from build123d import *

# Parameters (mm, degrees)
SKETCH1_W           = 38.481
SKETCH1_H           = 38.481
BOSS_EXTRUDE1_DEPTH = 12.573
SKETCH2_W           = 36.703
SKETCH2_H           = 36.703
CUT_EXTRUDE1_DEPTH  = 56.853872301
SKETCH3_R           = 2.4765
CUT_EXTRUDE2_DEPTH  = 55.644102143


with BuildPart() as part:
    # Sketch1 → Boss-Extrude1 (new body)
    with BuildSketch(Plane.XY):
        with Locations((19.2405, 19.2405)):
            Rectangle(SKETCH1_W, SKETCH1_H)
    extrude(amount=BOSS_EXTRUDE1_DEPTH)

    # Sketch2 → Cut-Extrude1 (cut, through all)
    with BuildSketch(Plane.XY.offset(12.573)):
        with Locations((18.3515, 20.1295)):
            Rectangle(SKETCH2_W, SKETCH2_H)
    extrude(amount=-CUT_EXTRUDE1_DEPTH, mode=Mode.SUBTRACT)

    # Sketch3 → Cut-Extrude2 (cut, through all)
    with BuildSketch(Plane.ZY.offset(-36.703)):
        with Locations(Location((6.2865, 12.6365, 0), (0, 0, 270))):
            Circle(SKETCH3_R)
        with Locations(Location((6.2865, 30.5435, 0), (0, 0, 270))):
            Circle(SKETCH3_R)
    cut_extrude2 = extrude(amount=-CUT_EXTRUDE2_DEPTH, mode=Mode.SUBTRACT)

    # Mirror1: Cut-Extrude2 across plane
    add(cut_extrude2.mirror(Plane(origin=(19.2405, 19.2405, 0), x_dir=(0, 0, 1), z_dir=(0.7071067811865389, 0.7071067811865561, 0))), mode=Mode.SUBTRACT)


solid = part.part
Verification items for the finished model (mm, model axes). A direction names the side the tool comes from. Coordinates: 2 decimals unless noted, no trailing zeros. Order: outer loops, then holes, each group sorted by start corner. A loop starts at its lowest first (then second) coordinate and runs counter-clockwise, first axis right, second up. Notation, with made-up numbers: (30, -0.75) -> (83, -0.75) arc R14 cw to (83, 16.25) -> close; hole circle Ø2 at (-5, 6.25). An arc over 180 degrees is marked (long way). Use CSV: the item, a comma, the result in double quotes. Start each with the question number.
Q1. Tool access check on faces 5 (the flat face through (18, 1.778, 6)), 6 (the cylindrical face through (37.58, 15.11, 6.4)). Record the directions out of +Z, -Z, +X, -X, +Y, -Y that give a thin tool (end or side, any length) a straight path to the whole face; none if there is none.
Q2. Thickness scan on line 1 along X through (y, z) = (10, 5.75); line 2 along Y through (x, z) = (23, 9.25). Record the ranges inside material, lowest first.
Q3. Section check B-B, the plane x = 8.5. Record the cut outline in (y, z), and give its area (3 significant figures).
Q4. Depth check by flat-ended pin: P1, Ø3, axis at x = 28, z = 9, coming from the +Y side. Enter the tip coordinate at first touch or a pass-through.
Q5. Section check C-C, the plane y = 31.5. Record the cut outline in (x, z), and give its area (3 significant figures).
Q6. Draft check along X on faces 1 (the flat face through (19, 0, 6)), 2 (the flat face through (38.481, 19, 6)), 3 (the cylindrical face through (5.97, 0.9, 4.78)), 4 (the cylindrical face through (28.207, 0.901, 7.03)). Enter one of: +X half, -X half, draft (parallel to the pull), parting line (faces both ways), or undercut.
Q7. Section check A-A, the plane z = 7. Record the cut outline in (x, y) (3 decimals), and give its area (3 significant figures).
Q8. Section check D-D, the plane z = 2.75. Record the cut outline in (x, y).
Returned:
1,face 5,"+Z, -Z, -X, +Y"
1,face 6,"+X, -X"
2,line 1,"x = 36.7 to 38.48"
2,line 2,"y = 0 to 1.78"
3,outline,"(0, 0) -> (1.78, 0) -> (1.78, 3.87) -> (0, 3.87) -> close; (0, 8.7) -> (1.78, 8.7) -> (1.78, 12.57) -> (0, 12.57) -> close"
3,area,"13.8 mm^2"
4,P1,"stops at y = 1.78"
5,outline,"(36.7, 0) -> (38.48, 0) -> (38.48, 4) -> (36.7, 4) -> close; (36.7, 8.57) -> (38.48, 8.57) -> (38.48, 12.57) -> (36.7, 12.57) -> close"
5,area,"14.2 mm^2"
6,face 1,"draft"
6,face 2,"+X half"
6,face 3,"undercut"
6,face 4,"undercut"
7,outline,"(0, 0) -> (5.566, 0) -> (5.566, 1.778) -> (0, 1.778) -> close; (10.309, 0) -> (23.473, 0) -> (23.473, 1.778) -> (10.309, 1.778) -> close; (28.216, 0) -> (38.481, 0) -> (38.481, 10.265) -> (36.703, 10.265) -> (36.703, 1.778) -> (28.216, 1.778) -> close; (36.703, 15.008) -> (38.481, 15.008) -> (38.481, 28.172) -> (36.703, 28.172) -> close; (36.703, 32.915) -> (38.481, 32.915) -> (38.481, 38.481) -> (36.703, 38.481) -> close"
7,area,"99.9 mm^2"
8,outline,"(0, 0) -> (38.48, 0) -> (38.48, 38.48) -> (36.7, 38.48) -> (36.7, 1.78) -> (0, 1.78) -> close"
